Geometry: final body of the model. Coordinates: model frame, mm. Face numbers are marked on the shaded views. A direction names the side the tool comes from. Round coordinates to 2 decimals unless told otherwise and drop trailing zeros. Loops run counter-clockwise (first coordinate to the right, second up) from the corner with the lowest first, then second, coordinate; pieces in that order, holes last. Notation, with made-up numbers: (-9, -27.75) - (12, -27.75) arc R31 cw to (12, 2.25) - close; hole circle Ø4 at (-11.5, 59.25). An arc over 180 degrees is marked (long way). Answer as CSV lines item,"result".
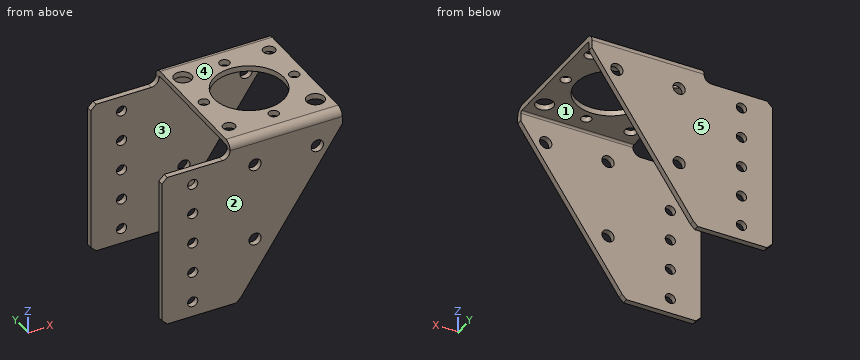
from build123d import *

# Parameters (mm, degrees)
SKETCH1_W                  = 42.545
SKETCH1_H                  = 50.927
BOSS_EXTRUDE1_DEPTH        = 6.2738
BOSS_EXTRUDE2_DEPTH        = 2.286
BOSS_EXTRUDE3_DEPTH        = 2.286
SKETCH4_W                  = 42.545
SKETCH4_H                  = 50.927
CUT_EXTRUDE1_DEPTH         = 3.9878
BOSS_EXTRUDE4_DEPTH        = 3.175
SKETCH6_W                  = 63.373
SKETCH6_H                  = 2.286
BOSS_EXTRUDE5_DEPTH        = 27.813
SKETCH7_W                  = 63.373
SKETCH7_H                  = 2.286
BOSS_EXTRUDE6_DEPTH        = 27.813
HOLE1_D                    = 4.9784
HOLE1_DEPTH                = 2.286
M3_5_CLEARANCE_HOLE1_D     = 4.1402
M3_5_CLEARANCE_HOLE1_DEPTH = 2.286
M25_CLEARANCE_HOLE1_D      = 28.575
M25_CLEARANCE_HOLE1_DEPTH  = 2.286025
HOLE2_D                    = 4.9784
HOLE2_DEPTH                = 2.286025
M6_5_CLEARANCE_HOLE1_D     = 7.1882
M6_5_CLEARANCE_HOLE1_DEPTH = 2.286025
M3_5_CLEARANCE_HOLE2_D     = 4.1402
M3_5_CLEARANCE_HOLE2_DEPTH = 2.286025
HOLE3_D                    = 4.9784
HOLE3_DEPTH                = 55.499
M3_5_CLEARANCE_HOLE3_D     = 4.1402
M3_5_CLEARANCE_HOLE3_DEPTH = 55.499
CHAMFER1_SIZE              = 2.159
CHAMFER1_SIZE2             = 0.59078994
CHAMFER2_SIZE              = 2.159
CHAMFER3_SIZE2             = 0.59078994
CHAMFER3_SIZE              = 2.159
FILLET1_R                  = 0.8128
FILLET2_R                  = 3.0988
FILLET3_R                  = 3.2004


with BuildPart() as part:
    # Sketch1 → Boss-Extrude1 (new body)
    with BuildSketch(Plane.XY.offset(2.286)):
        with Locations((1.5875, 0)):
            Rectangle(SKETCH1_W, SKETCH1_H)
    extrude(amount=-BOSS_EXTRUDE1_DEPTH)

    # Sketch2 → Boss-Extrude2 (add)
    with BuildSketch(Plane.XZ.offset(25.4635)):
        Polygon((-19.685, 2.286), (22.86, 2.286), (22.86, -3.9878), (-19.685, -67.437), align=None)
    extrude(amount=BOSS_EXTRUDE2_DEPTH)

    # Sketch3 → Boss-Extrude3 (add)
    with BuildSketch(Plane(origin=(0, 25.4635, 0), x_dir=(-1, 0, 0), z_dir=(0, 1, 0))):
        Polygon((19.685, -67.437), (-22.86, -3.9878), (-22.86, 2.286), (19.685, 2.286), align=None)
    extrude(amount=BOSS_EXTRUDE3_DEPTH)

    # Sketch4 → Cut-Extrude1 (cut)
    with BuildSketch(Plane(origin=(0, 0, -3.9878), x_dir=(-1, 0, 0), z_dir=(0, 0, -1))):
        with Locations((-1.5875, 0)):
            Rectangle(SKETCH4_W, SKETCH4_H)
    extrude(amount=-CUT_EXTRUDE1_DEPTH, mode=Mode.SUBTRACT)

    # Sketch5 → Boss-Extrude4 (add)
    with BuildSketch(Plane.ZY.offset(19.685)):
        Polygon((0, -25.4635), (0, 25.4635), (-67.437, 25.4635), (-67.437, 27.7495), (2.286, 27.7495), (2.286, -27.7495), (-67.437, -27.7495), (-67.437, -25.4635), align=None)
    extrude(amount=BOSS_EXTRUDE4_DEPTH)

    # Sketch6 → Boss-Extrude5 (add)
    with BuildSketch(Plane.ZY.offset(22.86)):
        with Locations((-35.7505, 26.6065)):
            Rectangle(SKETCH6_W, SKETCH6_H)
    extrude(amount=BOSS_EXTRUDE5_DEPTH)

    # Sketch7 → Boss-Extrude6 (add)
    with BuildSketch(Plane.ZY.offset(22.86)):
        with Locations((-35.7505, -26.6065)):
            Rectangle(SKETCH7_W, SKETCH7_H)
    extrude(amount=BOSS_EXTRUDE6_DEPTH)

    # Hole1
    with Locations(Plane(origin=(0, -25.4635, 0), x_dir=(1, 0, 0), z_dir=(0, 1, 0))):
        with Locations((-12.7, 10.1854), (12.7, 10.1854), (-12.7, 42.3164)):
            Hole(HOLE1_D / 2, depth=HOLE1_DEPTH)

    # M3.5 Clearance Hole1
    with Locations(Plane(origin=(0, -25.4635, 0), x_dir=(1, 0, 0), z_dir=(0, 1, 0))):
        with Locations((-38.1, 61.214), (-38.1, 48.514), (-38.1, 35.814), (-38.1, 23.114), (-38.1, 10.414)):
            Hole(M3_5_CLEARANCE_HOLE1_D / 2, depth=M3_5_CLEARANCE_HOLE1_DEPTH)

    # M25 Clearance Hole1
    with Locations(Plane(origin=(0, 0, 0), x_dir=(-1, 0, 0), z_dir=(0, 0, -1))):
        with Locations((0, 0)):
            Hole(M25_CLEARANCE_HOLE1_D / 2, depth=M25_CLEARANCE_HOLE1_DEPTH)

    # Hole2
    with Locations(Plane(origin=(0, 0, 0), x_dir=(-1, 0, 0), z_dir=(0, 0, -1))):
        with Locations((-17.960512242, 17.960512242), (17.960512242, -17.960512242)):
            Hole(HOLE2_D / 2, depth=HOLE2_DEPTH)

    # M6.5 Clearance Hole1
    with Locations(Plane(origin=(0, 0, 0), x_dir=(-1, 0, 0), z_dir=(0, 0, -1))):
        with Locations((17.5, 17.5), (-17.5, -17.5)):
            Hole(M6_5_CLEARANCE_HOLE1_D / 2, depth=M6_5_CLEARANCE_HOLE1_DEPTH)

    # M3.5 Clearance Hole2
    with Locations(Plane(origin=(0, 0, 0), x_dir=(-1, 0, 0), z_dir=(0, 0, -1))):
        with Locations((18.415, 0), (0, 18.415), (0, -18.415), (-18.415, 0)):
            Hole(M3_5_CLEARANCE_HOLE2_D / 2, depth=M3_5_CLEARANCE_HOLE2_DEPTH)

    # Hole3
    with Locations(Plane(origin=(0, 27.7495, 0), x_dir=(1, 0, 0), z_dir=(0, 1, 0))):
        with Locations((-12.7, 10.1854), (12.7, 10.1854), (-12.7, 42.3164)):
            Hole(HOLE3_D / 2, depth=HOLE3_DEPTH)

    # M3.5 Clearance Hole3
    with Locations(Plane(origin=(0, 27.7495, 0), x_dir=(1, 0, 0), z_dir=(0, 1, 0))):
        with Locations((-38.1, 61.214), (-38.1, 48.514), (-38.1, 35.814), (-38.1, 23.114), (-38.1, 10.414)):
            Hole(M3_5_CLEARANCE_HOLE3_D / 2, depth=M3_5_CLEARANCE_HOLE3_DEPTH)

    # Chamfer1
    chamfer1_edges = [part.edges().sort_by_distance(p)[0] for p in [
        (-19.685, -26.6065, -67.437),
    ]]
    chamfer1_side = [part.faces().sort_by_distance(p)[0] for p in [
        (1.5875, -26.6065, -35.7124),
    ]]
    chamfer(chamfer1_edges, length=CHAMFER1_SIZE, length2=CHAMFER1_SIZE2, reference=chamfer1_side[0])

    # Chamfer2
    chamfer2_edges = [part.edges().sort_by_distance(p)[0] for p in [
        (-50.673, -26.6065, -67.437),
        (-50.673, 26.6065, -67.437),
        (-50.673, -26.6065, -4.064),
        (-50.673, 26.6065, -4.064),
    ]]
    chamfer(chamfer2_edges, length=CHAMFER2_SIZE)

    # Chamfer3
    chamfer3_edges = [part.edges().sort_by_distance(p)[0] for p in [
        (-19.685, 26.6065, -67.437),
    ]]
    chamfer(chamfer3_edges, length=CHAMFER3_SIZE, length2=CHAMFER3_SIZE2)

    # Fillet1
    fillet1_edges = [part.edges().sort_by_distance(p)[0] for p in [
        (0, 25.4635, 0),
        (0, -25.4635, 0),
    ]]
    fillet(fillet1_edges, radius=FILLET1_R)

    # Fillet2
    fillet2_edges = [part.edges().sort_by_distance(p)[0] for p in [
        (0, 27.7495, 2.286),
        (0, -27.7495, 2.286),
    ]]
    fillet(fillet2_edges, radius=FILLET2_R)

    # Fillet3
    fillet3_edges = [part.edges().sort_by_distance(p)[0] for p in [
        (-22.86, 26.6065, -4.064),
        (-22.86, -26.6065, -4.064),
    ]]
    fillet(fillet3_edges, radius=FILLET3_R)


solid = part.part
(1) Section C-C (z = -27). Output: boundary loops of the cut face in (x, y).
Findings below:
outline,"(-50.67, -27.75) - (7.43, -27.75) - (7.43, -25.46) - (-50.67, -25.46) - close; (-50.67, 25.46) - (7.43, 25.46) - (7.43, 27.75) - (-50.67, 27.75) - close"
(2) Draft query along Y for the marked faces 3, 4 and 5. Return one class per face: pulls with the +Y half, pulls with the -Y half, needs draft (parallel to the pull), parting line crosses it, or undercut.
Findings below:
face 3,"undercut"
face 4,"needs draft"
face 5,"pulls with the +Y half"
(3) Section A-A (y = 0). Output: boundary loops of the cut face in (x, z), and give its area (3 significant figures).
Findings below:
outline,"(-22.86, 0) - (-20.49, 0) - (-20.49, 2.29) - (-22.86, 2.29) - close; (-16.34, 0) - (-14.29, 0) - (-14.29, 2.29) - (-16.34, 2.29) - close; (14.29, 0) - (16.34, 0) - (16.34, 2.29) - (14.29, 2.29) - close; (20.49, 0) - (22.86, 0) - (22.86, 2.29) - (20.49, 2.29) - close"
area,"20.3 mm2"
(4) Section D-D (y = 11). Output: boundary loops of the cut face in (x, z).
Findings below:
outline,"(-22.86, 0) - (-9.12, 0) - (-9.12, 2.29) - (-22.86, 2.29) - close; (9.12, 0) - (22.86, 0) - (22.86, 2.29) - (9.12, 2.29) - close"
(5) Pin query (flat end, axial travel): P1, Ø8, axis at x = 17.96, y = 17.96, coming from the -Z side; P2, Ø1.1, axis at x = -35.5, y = -27, coming from the +Z side; P3, Ø3.5, axis at x = 0, y = -18.415, coming from the -Z side; P4, Ø3.5, axis at y = -10.5, z = 0.5, coming from the -X side. Return the tip coordinate at first contact, or that it passes through.
Findings below:
P1,"z = 0"
P2,"z = -4.06"
P3,"through"
P4,"x = -22.86"
(6) Section B-B (x = 17.5). Output: boundary loops of the cut face in (y, z), and give its area (3 significant figures).
Findings below:
outline,"(-27.75, -11.98) - (-25.46, -11.98) - (-25.46, -0.81) arc R0.81 cw to (-24.65, 0) - (-21.09, 0) - (-21.09, 2.29) - (-24.65, 2.29) arc R3.1 ccw to (-27.75, -0.81) - close; (-13.91, 0) - (-1.86, 0) - (-1.86, 2.29) - (-13.91, 2.29) - close; (1.86, 0) - (15.51, 0) - (15.51, 2.29) - (1.86, 2.29) - close; (20.41, 0) - (24.65, 0) arc R0.81 cw to (25.46, -0.81) - (25.46, -11.98) - (27.75, -11.98) - (27.75, -0.81) arc R3.1 ccw to (24.65, 2.29) - (20.41, 2.29) - close"
area,"142 mm2"
(7) Material intervals for line 1 along Z through (x, y) = (-38.1, 27.2); line 2 along Y through (x, z) = (-30.5, -35.5); line 3 along Y through (x, z) = (0, 0.75), sorted ascending.
Findings below:
line 1,"-67.44 to -63.28, -59.14 to -50.58, -46.44 to -37.88, -33.74 to -25.18, -21.04 to -12.48, -8.34 to -4.06"
line 2,"-27.75 to -25.46, 25.46 to 27.75"
line 3,"-27.33 to -20.49, -16.34 to -14.29, 14.29 to 16.34, 20.49 to 27.33"
(8) Access query for the marked faces 1 and 2. Directions: +Z, -Z, +X, -X, +Y, -Y. A direction counts if a zero-diameter tool reaches every point of the face in a straight line with its end or side. Return the directions, or none.
Findings below:
face 1,"-Z, +X, -X"
face 2,"+Z, -Z, +X, -X, -Y"
